Print and shaded views of the part. All mm, measured from the part's lowest x, y and z. A direction names the side the tool comes from. Round coordinates to 2 decimals unless told otherwise and drop trailing zeros. Loops run counter-clockwise (first coordinate to the right, second up) from the corner with the lowest first, then second, coordinate; pieces in that order, holes last. Notation, with made-up numbers: (36, 42) -> (84, 42) arc R24 ccw to (84, 70) -> close; hole circle Ø1 at (63.5, 62). An arc over 180 degrees is marked (long way). Use a Markdown table: item, result.
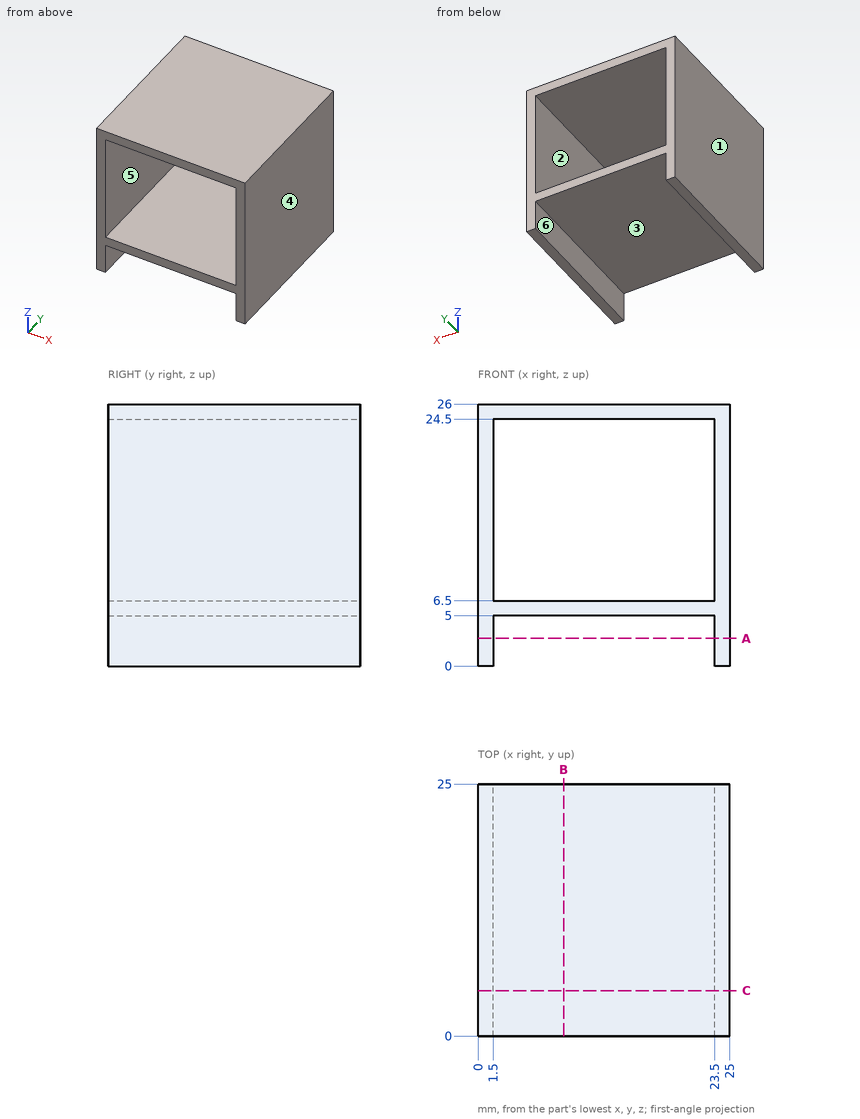
Q1. Band-saw the part on A-A, the plane z = 2.75. Give the cut face in (x, y).
Results list:
| item | result |
|---|---|
| outline | (0, 0) -> (1.5, 0) -> (1.5, 25) -> (0, 25) -> close; (23.5, 0) -> (25, 0) -> (25, 25) -> (23.5, 25) -> close |
Q2. Tool access for the marked faces 4, 5 and 6: list every direction of +Z, -Z, +X, -X, +Y, -Y with a clear straight run to the whole face (end or side of a thin tool).
Results list:
| item | result |
|---|---|
| face 4 | +Z, -Z, +X, +Y, -Y |
| face 5 | +Y, -Y |
| face 6 | -Z, +Y, -Y |
Q3. Band-saw the part on B-B, the plane x = 8.5. Give the cut face in (y, z), plus the area to 3 significant figures.
Results list:
| item | result |
|---|---|
| outline | (0, 5) -> (25, 5) -> (25, 6.5) -> (0, 6.5) -> close; (0, 24.5) -> (25, 24.5) -> (25, 26) -> (0, 26) -> close |
| area | 75.0 mm² |
Q4. Drill centre lines: L1, parallel to Z at x = 10.25, y = 15; L2, parallel to X at y = 1, z = 4. Where is each one in solid material? Low to high. Write a range as from..to.
Results list:
| item | result |
|---|---|
| L1 | z = 5..6.5, 24.5..26 |
| L2 | x = 0..1.5, 23.5..25 |
Q5. Pull direction Z, two halves, no side cores. Call the marked faces 1, 2 and 3: released by +Z, released by -Z, zero draft, split by the parting line, or undercut.
Results list:
| item | result |
|---|---|
| face 1 | zero draft |
| face 2 | undercut |
| face 3 | released by -Z |
Q6. Band-saw the part on C-C, the plane y = 4.5. Give the cut face in (x, z).
Results list:
| item | result |
|---|---|
| outline | (0, 0) -> (1.5, 0) -> (1.5, 5) -> (23.5, 5) -> (23.5, 0) -> (25, 0) -> (25, 26) -> (0, 26) -> close; hole (1.5, 6.5) -> (23.5, 6.5) -> (23.5, 24.5) -> (1.5, 24.5) -> close |
Q7. Flat gauge pin, fed straight in: pin 1 (1.5 mm diameter, centred on x = 14.5, z = 3.5, fed in from -Y). Where does the tip first touch, or does it go through?
Results list:
| item | result |
|---|---|
| pin 1 | passes through |
